Part print with two shaded views. Sizes in mm from the minimum x, y, z corner. Give positions to 0.01 mm unless a question says otherwise; leave off trailing zeros. Loops run counter-clockwise (first coordinate to the right, second up) from the corner with the lowest first, then second, coordinate; pieces in that order, holes last. Notation, with made-up numbers: (-23.5, 29.5) -> (-3.5, 29.5) arc R17 ccw to (-3.5, 57.5) -> close; hole circle Ø5 at (-2.5, -7.75). An arc over 180 degrees is marked (long way). One line per question, with ' | ' between items. Start each with the question number.
(1) Slice it at B-B, the plane y = 2.5. Give the number of separate pieces and of enclosed holes in the cut face, then the cut area to 3 significant figures.
(2) Slice it at C-C, the plane z = 50. Write the cut outline in (x, y) (1 decimal), then the cut area to 3 significant figures.
(3) Slice it at D-D, the plane x = 23.5. Write the cut outline in (y, z) (1 decimal).
(4) Slice it at A-A, the plane z = 85.94. Write the cut outline in (x, y) (1 decimal).
(5) Flat gauge pins, fed straight in: pin 1 Ø5 at (x, z) = (76.27, 50) entering from -Y; pin 2 Ø1 at (y, z) = (2, 79) entering from -X (1 decimal). Where does each tip first touch, or does it go through?
(6) Drill centre lines: L1, parallel to Z at x = 66.5, y = 0.9; L2, parallel to X at y = 1.5, z = 98.69 (1 decimal); L3, parallel to X at y = 2.4, z = 50 (1 decimal). Where is each one in solid material? Low to high. Write a range as from..to.
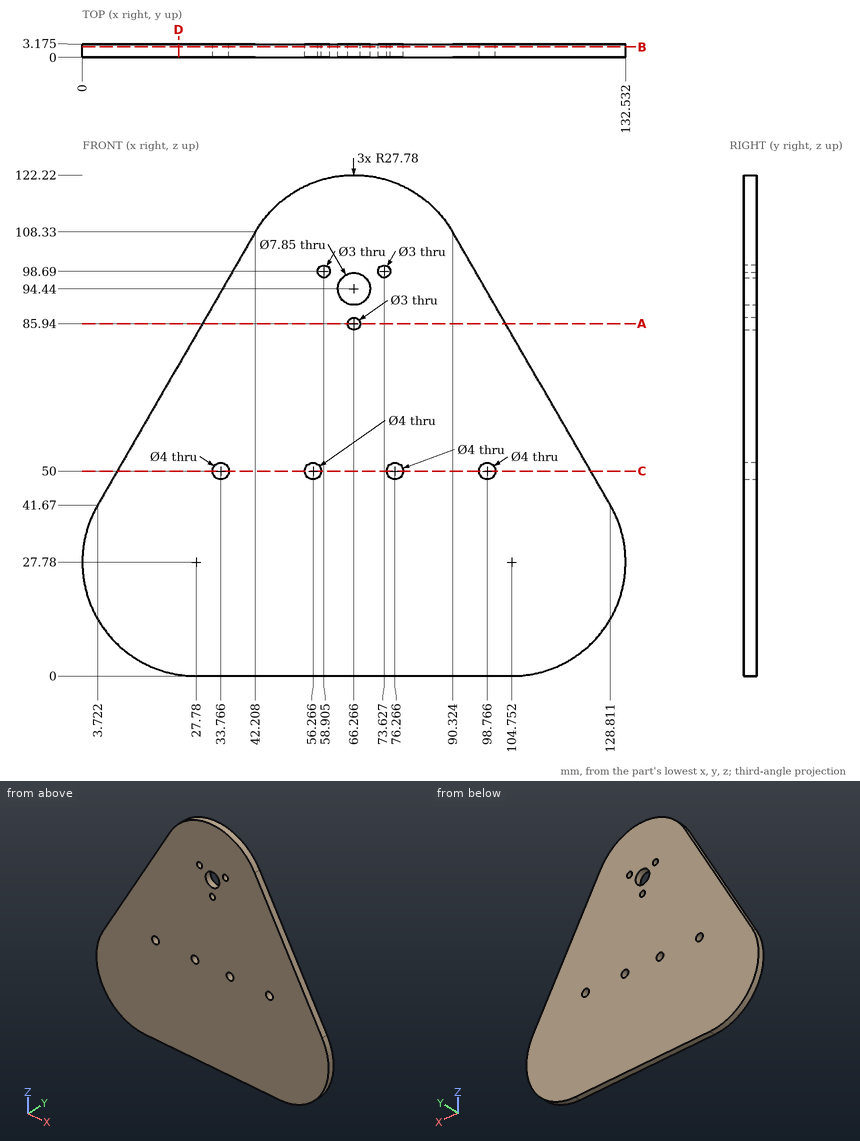
Final values:
1) separate pieces: 1 | enclosed holes: 8 | area: 11,300 mm2
2) outline: (8.5, 0) -> (31.8, 0) -> (31.8, 3.2) -> (8.5, 3.2) -> close; (35.8, 0) -> (54.3, 0) -> (54.3, 3.2) -> (35.8, 3.2) -> close; (58.3, 0) -> (74.3, 0) -> (74.3, 3.2) -> (58.3, 3.2) -> close; (78.3, 0) -> (96.8, 0) -> (96.8, 3.2) -> (78.3, 3.2) -> close; (100.8, 0) -> (124, 0) -> (124, 3.2) -> (100.8, 3.2) -> close | area: 316 mm2
3) outline: (0, 0.3) -> (3.2, 0.3) -> (3.2, 75.9) -> (0, 75.9) -> close
4) outline: (29.3, 0) -> (64.8, 0) -> (64.8, 3.2) -> (29.3, 3.2) -> close; (67.8, 0) -> (103.3, 0) -> (103.3, 3.2) -> (67.8, 3.2) -> close
5) pin 1: y = 0 | pin 2: x = 25
6) L1: 0..84.46, 87.42..90.52, 98.36..122.22 | L2: 36.6..57.4, 60.4..72.1, 75.1..95.9 | L3: 8.5..31.8, 35.8..54.3, 58.3..74.3, 78.3..96.8, 100.8..124
